Model file for the job. Use its own axes, mm. A direction names the side the tool comes from. Give positions to 0.01 mm unless a question says otherwise; leave off trailing zeros. Loops run counter-clockwise (first coordinate to the right, second up) from the corner with the lowest first, then second, coordinate; pieces in that order, holes last. Notation, with made-up numbers: (-11.5, 18) - (45.5, 18) arc R30 ccw to (45.5, 45) - close; hole circle Ø5 at (78, -10.75). An arc over 180 degrees is marked (long way). Answer as CSV lines item,"result". Start each with the question number.
Item 1: Saw through at C-C on z = -83. Give the cut face in (x, y), plus the area to 3 significant figures.
Item 2: Pull direction Y, two halves, no side cores. Call faces 4 (the flat face through (-237, -1.588, -89)), 5 (the flat face through (-243, 61, 0)), 6 (the flat face through (-231.45, 12.51, 0.78)): pulls with the +Y half, pulls with the -Y half, needs draft (parallel to the pull), parting line crosses it, or undercut.
Item 3: Pin check, flat tips, straight feed: pin 1 (0.5 mm diameter, centred on y = 69, z = 0.5, fed in from +X); pin 2 (4 mm diameter, centred on x = -239, z = -67, fed in from +Y); pin 3 (5 mm diameter, centred on y = 1, z = -52.5, fed in from +X). Stop position of each tip, or through.
Item 4: Saw through at A-A on x = -231. Give the cut face in (y, z).
Item 5: Saw through at D-D on x = -245. Give the cut face in (y, z).
Item 6: Tool access for faces 1 (the flat face through (-237, 0, -89)), 2 (the flat face through (-231, 108, 1)), 3 (the cylindrical face through (-236.739, 111.036, 0.783)): list every direction of +Z, -Z, +X, -X, +Y, -Y with a clear straight run to the whole face (end or side of a thin tool).
Item 7: Saw through at B-B on y = 97.5. Give the cut face in (x, z), plus the area to 3 significant figures.
Item 8: Drill centre lines: L1, parallel to Y at x = -237.5, z = 1; L2, parallel to Z at x = -241, y = 87; L3, parallel to Y at x = -248.25, z = -80. Where is each one in solid material? Low to high. Write a range as from..to.
from build123d import *

# Parameters (mm, degrees)
SKETCH1_R           = 1.65
BOSS_EXTRUDE1_DEPTH = 1.5875
SKETCH2_W           = 25.4
SKETCH2_H           = 177.8
BOSS_EXTRUDE2_DEPTH = 1.5875


with BuildPart() as part:
    # Sketch1 → Boss-Extrude1 (new body)
    with BuildSketch(Plane.XY):
        Polygon((-223.5, 120), (-250, 120), (-250, 0), (-224.6, 0), (-224.6, 4.746666667), (-238.5, 20.5), (-238.5, 99.5), (-223.5, 116.5), align=None)
        with Locations((-237.5, 7.5)):
            Circle(SKETCH1_R, mode=Mode.SUBTRACT)
        with Locations((-237.5, 112.5)):
            Circle(SKETCH1_R, mode=Mode.SUBTRACT)
    extrude(amount=BOSS_EXTRUDE1_DEPTH)

    # Sketch2 → Boss-Extrude2 (add)
    with BuildSketch(Plane(origin=(0, 0, 0), x_dir=(1, 0, 0), z_dir=(0, 1, 0))):
        with Locations((-237.3, 87.3125)):
            Rectangle(SKETCH2_W, SKETCH2_H)
    extrude(amount=-BOSS_EXTRUDE2_DEPTH)


solid = part.part
Responses:
1,outline,"(-250, -1.59) - (-224.6, -1.59) - (-224.6, 0) - (-250, 0) - close"
1,area,"40.3 mm2"
2,face 4,"pulls with the -Y half"
2,face 5,"needs draft"
2,face 6,"undercut"
3,pin 1,"x = -238.5"
3,pin 2,"y = 0"
3,pin 3,"x = -224.6"
4,outline,"(-1.59, -176.21) - (0, -176.21) - (0, 0) - (12, 0) - (12, 1.59) - (-1.59, 1.59) - close; (108, 0) - (120, 0) - (120, 1.59) - (108, 1.59) - close"
5,outline,"(-1.59, -176.21) - (0, -176.21) - (0, 0) - (120, 0) - (120, 1.59) - (-1.59, 1.59) - close"
6,face 1,"-Z, +X, -X, +Y"
6,face 2,"+Z, -Z, +X"
6,face 3,"+Z, -Z"
7,outline,"(-250, 0) - (-238.5, 0) - (-238.5, 1.59) - (-250, 1.59) - close"
7,area,"18.3 mm2"
8,L1,"-1.59..5.85, 9.15..19.37, 100.63..110.85, 114.15..120"
8,L2,"0..1.59"
8,L3,"-1.59..0"
